Could you check a few things on this model? Use its own coordinates, in mm. A direction names the side the tool comes from. Round coordinates to 2 decimals unless told otherwise and drop trailing zeros. Write each loop counter-clockwise with the first axis right and the second up, starting at its lowest first coordinate (ties: lowest second). Pieces come first, ordered by that corner, then holes. Notation, with made-up numbers: (88.25, 31.5) - (143.25, 31.5) arc R21 cw to (143.25, 67.5) - close; hole circle Ø1 at (-22.5, -38.5). An arc over 180 degrees is marked (long way). Write each question's results on one line, items separated by ' | '. Start each with the question number.
(1) Imagine slicing it at B-B on x = 5. Write out the boundary of the cut face in (y, z).
(2) Imagine slicing it at D-D on z = 20.5. Write out the boundary of the cut face in (x, y).
(3) Please list where these lines run through material, in increasing order: line 1 (X direction, y = 0, z = 20.5); line 2 (X direction, y = 0, z = 12.5). Write a range as [from, to].
(4) Imagine slicing it at A-A on y = 0. Write out the boundary of the cut face in (x, z), then the cut area to 3 significant figures.
(5) For P1, Ø8, axis at y = -8, z = 13.5, coming from the -X side; P2, Ø3, axis at x = -13.5, z = 26, coming from the -Y side; P3, Ø3, axis at x = -8.5, y = -18.5, coming from the -Z side; P4, Ø6, axis at x = -11, y = 4.5, coming from the -Z side, each with a flat end and sliding along its axis, tell me the tip position at first contact or that it passes through.
(6) On a 3-axis mill with a long thin cutter (end or side, diameter ignored), from which of +Z, -Z, +X, -X, +Y, -Y can I reach the whole of each face in a straight line? I mean faces 1 (the flat face through (54, -8, 14)), 2 (the flat face through (54, -12, 12)), 3 (the flat face through (43, 4, 6)), 4 (the flat face through (16, 0, 24)), 5 (the cylindrical face through (66, 0, 10)). Say none if no direction works.
(7) Thinking about a two-plate mould opening in X: for faces 6 (the flat face through (-17, 0, 24)), 7 (the cylindrical face through (36, 0, 12)), which applies, +X half, -X half, draft (parallel to the pull), parting line (faces both ways), or undercut?
(8) Imagine slicing it at C-C on y = 9. Write out the boundary of the cut face in (x, z).
Autodesk Inventor part; units mm, degrees
ref_plane "Arbeitsebene2" through (85, 0, 0) normal (1, 0, 0) x (0, 1, 0)
ref_plane "XZ Plane" through (0, 0, 0) normal (0, 1, 0) x (-1, 0, 0)
ref_plane "XY Plane" through (0, 0, 0) normal (0, 0, 1) x (1, 0, 0)
sketch "Skizze1" plane through (0, 0, 0) normal (0, 0, 1) x (1, 0, 0)
  line L0 (0, 25) -> (60, 25)
  line L1 (0, -25) -> (60, -25)
  circle A0 centre (0, 0) radius 25
  arc A1 (60, -25) -> (60, 25) centre (60, 0) ccw
  line L2 (0, 0) -> (60, 0) construction
  point P0 (0, 0)
  dimension "d1" = 25
  dimension "d2" = 50
  dimension "d3" = 60
extrude "Extrusion1" add sketch "Skizze1" along normal blind 10 contours L0 A1 L1 A0
extrude "Extrusion2" add sketch "Skizze1" along normal blind 30 contours A0
sketch "Skizze3" plane through (0, 0, 30) normal (0, 0, 1) x (1, 0, 0)
  circle A0 centre (0, 0) radius 25
  line L0 (-24.2693, 6) -> (24.2693, 6)
  line L1 (-24.2693, -6) -> (24.2693, -6)
  line L2 (-25, 0) -> (25, 0) construction
  point P0 (0, 0)
  point P1 (0, 0)
  dimension "d11" = 12
extrude "Extrusion4" cut sketch "Skizze3" against normal blind 6 contours A0 L1 L0
sketch "Skizze4" plane through (0, 0, 30) normal (0, 0, 1) x (1, 0, 0)
  circle A0 centre (0, 0) radius 10
  dimension "d14" = 20
extrude "Extrusion5" cut sketch "Skizze4" against normal up to surface (30 mm away)
sketch "Skizze5" plane through (0, 0, 10) normal (0, 0, 1) x (1, 0, 0)
  line L0 (48, 0) -> (60, 0) construction
  line L1 (48, -6) -> (60, -6)
  line L2 (60, 6) -> (48, 6)
  arc A0 (48, 6) -> (48, -6) centre (48, 0) ccw
  arc A1 (60, -6) -> (60, 6) centre (60, 0) ccw
  line L3 (48, 0) -> (60, 0) construction
  line L4 (48, -12) -> (60, -12)
  line L5 (60, 12) -> (48, 12)
  arc A2 (48, 12) -> (48, -12) centre (48, 0) ccw
  arc A3 (60, -12) -> (60, 12) centre (60, 0) ccw
  point P0 (0, 0)
  point P1 (54, 0)
  point P2 (54, 0)
  dimension "d17" = 12
  dimension "d18" = 60
  dimension "d19" = 6
  dimension "d20" = 12
extrude "Extrusion6" cut sketch "Skizze5" against normal up to surface (10 mm away) contours A0 L2 A1 L1
extrude "Extrusion7" add sketch "Skizze5" along normal blind 4
ref_plane "Arbeitsebene2" through (85, 0, 0) normal (1, 0, 0) x (0, 1, 0)
sketch "Skizze6" plane through (85, 0, 0) normal (1, 0, 0) x (0, 1, 0)
  line L0 (25, 0) -> (-25, 0)
  line L1 (-10, 0) -> (-10, 6)
  line L2 (-10, 6) -> (10, 6)
  line L3 (10, 6) -> (10, -0.2109)
  line L4 (0, 0) -> (0, 8.6058) construction
  line L5 (25, 10) -> (-25, 10)
  point P0 (0, 6)
  point P1 (0, 10)
  point P2 (10, 0)
  dimension "d26" = 20
  dimension "d27" = 4
extrude "Extrusion8" cut sketch "Skizze6" against normal through all
properties part number "slider" material "Stahl, galvanisiert"
Response:
1) outline: (-25, 0) - (-10, 0) - (-10, 6) - (-8.66, 6) - (-8.66, 30) - (-24.49, 30) - (-24.49, 10) - (-25, 10) - close; (8.66, 6) - (10, 6) - (10, 0) - (25, 0) - (25, 10) - (24.49, 10) - (24.49, 30) - (8.66, 30) - close
2) outline: circle Ø50 at (0, 0); hole circle Ø20 at (0, 0)
3) line 1: [-25, -10], [10, 25] | line 2: [-25, -10], [10, 25], [36, 42], [66, 72]
4) outline: (-25, 6) - (-10, 6) - (-10, 24) - (-25, 24) - close; (10, 6) - (42, 6) - (42, 14) - (36, 14) - (36, 10) - (25, 10) - (25, 24) - (10, 24) - close; (66, 6) - (85, 6) - (85, 10) - (72, 10) - (72, 14) - (66, 14) - close | area: 732 mm²
5) P1: x = -24.68 | P2: y = -21.93 | P3: z = 0 | P4: z = 6
6) face 1: +Z, +X, +Y, -Y | face 2: +Z, +X, -Y | face 3: -Z, +X, -X | face 4: +Z, +X, -X | face 5: +Z, -Z
7) face 6: draft | face 7: undercut
8) outline: (-23.32, 6) - (-4.36, 6) - (-4.36, 30) - (-23.32, 30) - close; (4.36, 6) - (83.32, 6) - (83.32, 10) - (67.94, 10) - (67.94, 14) - (40.06, 14) - (40.06, 10) - (23.32, 10) - (23.32, 30) - (4.36, 30) - close
